The model under review builds one solid part; all positions refer to its coordinate system, in mm. Coordinates: 2 decimals unless noted, no trailing zeros. Write each loop counter-clockwise with the first axis right and the second up, starting at its lowest first coordinate (ties: lowest second). Pieces come first, ordered by that corner, then holes.
```python
from build123d import *

# Parameters (mm, degrees)
F0_R     = 1.25
F1_DEPTH = 5
F2_DEPTH = 5
F3_DEPTH = 5


with BuildPart() as f1:
    # F0 (on Top) → F1 (new body)
    with BuildSketch(Plane.XY):
        with BuildLine():
            ThreePointArc((52.175985, 23.970867), (10.978788, 30.890651), (-25.696786, 50.89052))
            ThreePointArc((-25.696786, 50.89052), (-161.829837, -1.114364), (-25.706141, -53.143729))
            ThreePointArc((-25.706141, -53.143729), (10.971628, -33.137817), (52.175985, -26.231581))
            Line((52.175985, -26.231581), (52.175985, -1.131581))
            Line((52.175985, -1.131581), (52.175985, 23.970867))
        make_face()
        with Locations((-83.827306, -76.123909)):
            Circle(F0_R, mode=Mode.SUBTRACT)
        with Locations((-158.829837, -1.128392)):
            Circle(F0_R, mode=Mode.SUBTRACT)
        with Locations((-83.827306, 73.881153)):
            Circle(F0_R, mode=Mode.SUBTRACT)
        with Locations((21.709267, -0.885356)):
            Circle(F0_R, mode=Mode.SUBTRACT)
        with Locations((39.925987, 19.149961)):
            Circle(F0_R, mode=Mode.SUBTRACT)
    extrude(amount=-F1_DEPTH)


with BuildPart() as f2:
    # F0 (on Top) → F2 (new body)
    with BuildSketch(Plane.XY):
        with Locations((39.925987, 19.149961)):
            Circle(F0_R)
        with Locations((21.709267, -0.885356)):
            Circle(F0_R)
        with Locations((-83.827306, 73.881153)):
            Circle(F0_R)
        with Locations((-83.827306, -76.123909)):
            Circle(F0_R)
        with Locations((-158.829837, -1.128392)):
            Circle(F0_R)
    extrude(amount=F2_DEPTH)


with BuildPart() as f3:
    # F0 (on Top) → F3 (new body)
    with BuildSketch(Plane.XY):
        with Locations((-158.829837, -1.128392)):
            Circle(F0_R)
        with Locations((-83.827306, -76.123909)):
            Circle(F0_R)
        with Locations((-83.827306, 73.881153)):
            Circle(F0_R)
        with Locations((21.709267, -0.885356)):
            Circle(F0_R)
        with Locations((39.925987, 19.149961)):
            Circle(F0_R)
    extrude(amount=-F3_DEPTH)


with BuildPart() as f1_1:
    add(f1.part)

    # F4: union F2, F3
    add(f2.part)
    add(f3.part)


solid = f1_1.part
```
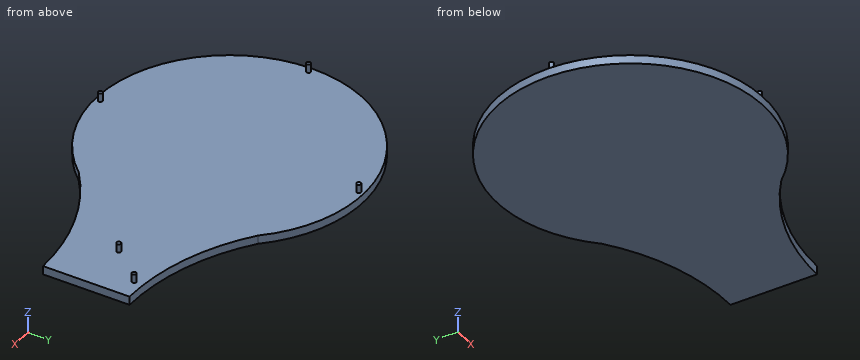
Item 1: To check wall thickness, follow line 1 along Z through (x, y) = (-29, -49); line 2 along X through (y, z) = (10, -1.5); line 3 along Y through (x, z) = (-124, -1.5). State the ranges of each line that lie inside material, in increasing order.
Solved:
line 1: z = -5 to 0
line 2: x = -161.03 to 52.18
line 3: y = -67.98 to 65.74
Item 2: Take a section at B-B, the plane x = -108.5. Write out the cut boundary in (y, z), plus the area to 3 significant figures.
Solved:
outline: (-75.12, -5) - (72.88, -5) - (72.88, 0) - (-75.12, 0) - close
area: 740 mm2
Item 3: Take a section at A-A, the plane z = -2.5. Write out the cut boundary in (x, y).
Solved:
outline: (-25.71, -53.14) arc R125.94 cw to (52.18, -26.23) - (52.18, 23.97) arc R126.09 cw to (-25.7, 50.89) arc R78 ccw (long way) to start
Item 4: For pin 1 (5 mm diameter, centred on x = -66.5, y = -22, fed in from +Z); pin 2 (6 mm diameter, centred on y = 21.5, z = -4, fed in from -X); pin 3 (2 mm diameter, centred on y = -16.5, z = 2, fed in from +X); pin 4 (1.5 mm diameter, centred on y = -53.5, z = -1, fed in from -X), all flat-tipped, find the tip position at first contact; note any pin that passes through.
Solved:
pin 1: stops at z = 0
pin 2: stops at x = -159.32
pin 3: passes through
pin 4: stops at x = -142.3
